Geometry check sheet. Reference: the model listing, model coordinates, mm. Coordinates: 2 decimals unless noted, no trailing zeros. Write each loop counter-clockwise with the first axis right and the second up, starting at its lowest first coordinate (ties: lowest second). Pieces come first, ordered by that corner, then holes.
from build123d import *

# Parameters (mm, degrees)
F0_W     = 30
F0_H     = 100
F0_R     = 10
F2_DEPTH = 30
F3_D     = 20


with BuildPart() as f2:
    # F0 (on Front) → F2 (new body)
    with BuildSketch(Plane.XZ):
        with Locations((15, 50)):
            Rectangle(F0_W, F0_H)
        with Locations((15, 25)):
            Circle(F0_R, mode=Mode.SUBTRACT)
    extrude(amount=-F2_DEPTH)

    # F3 (through all)
    with Locations(Plane(origin=(0, 0, 0), x_dir=(0, 1, 0), z_dir=(-1, 0, 0))):
        with Locations((15, -75)):
            Hole(F3_D / 2)


solid = f2.part
1. Sectioned sample at B-B, the plane x = 15. Record the boundary of the cut face in (y, z), and give its area (3 significant figures).
Computed values:
outline: (0, 0) - (30, 0) - (30, 15) - (0, 15) - close; (0, 35) - (30, 35) - (30, 100) - (0, 100) - close; hole circle Ø20 at (15, 75)
area: 2,090 mm2
2. Sectioned sample at D-D, the plane x = 27.25. Record the boundary of the cut face in (y, z), and give its area (3 significant figures).
Computed values:
outline: (0, 0) - (30, 0) - (30, 100) - (0, 100) - close; hole circle Ø20 at (15, 75)
area: 2,690 mm2
3. Sectioned sample at A-A, the plane y = 15. Record the boundary of the cut face in (x, z).
Computed values:
outline: (0, 0) - (30, 0) - (30, 65) - (0, 65) - close; (0, 85) - (30, 85) - (30, 100) - (0, 100) - close; hole circle Ø20 at (15, 25)
4. Sectioned sample at C-C, the plane z = 25. Record the boundary of the cut face in (x, y), and give its area (3 significant figures).
Computed values:
outline: (0, 0) - (5, 0) - (5, 30) - (0, 30) - close; (25, 0) - (30, 0) - (30, 30) - (25, 30) - close
area: 300 mm2
5. Draft check along Y on faces 1 (the flat face through (15, 30, 51)), 2 (the flat face through (15, 15, 100)), 3 (the flat face through (15, 0, 51)), 4 (the cylindrical face through (15.21, 9.62, 66.57)). Enter one of: released by +Y, released by -Y, zero draft, split by the parting line, or undercut.
Computed values:
face 1: released by +Y
face 2: zero draft
face 3: released by -Y
face 4: undercut
6. Gauge pin test, flat end, axial feed: pin 1 Ø18 at (x, z) = (15, 25) entering from -Y. Record the tip position at first contact, or that the pin passes through.
Computed values:
pin 1: passes through
7. Thickness scan on line 1 along Y through (x, z) = (16, 75); line 2 along Z through (x, y) = (6, 22.25); line 3 along Z through (x, y) = (20.75, 23.25). Record the ranges inside material, lowest first.
Computed values:
line 1: y = 0 to 5, 25 to 30
line 2: z = 0 to 20.64, 29.36 to 68.11, 81.89 to 100
line 3: z = 0 to 16.82, 33.18 to 69.35, 80.65 to 100
